from build123d import *

# Parameters (mm, degrees)
SZKIC1_R                    = 3
DODANIE_WYCI_GNI_CIE2_DEPTH = 2.4
SZKIC2_R                    = 1.5
DODANIE_WYCI_GNI_CIE3_DEPTH = 5
ZAOKR_GLENIE2_R             = 1.2
WYTNIJ_WYCI_GNI_CIE1_DEPTH  = 1.94


with BuildPart() as part:
    # Szkic1 → Dodanie-wyciągnięcie2 (new body)
    with BuildSketch(Plane.XY):
        with Locations((-1.860516246, 2.732142857)):
            Circle(SZKIC1_R)
    extrude(amount=DODANIE_WYCI_GNI_CIE2_DEPTH)

    # Szkic2 → Dodanie-wyciągnięcie3 (add)
    with BuildSketch(Plane(origin=(0, 0, 0), x_dir=(-1, 0, 0), z_dir=(0, 0, -1))):
        with Locations((1.860516246, 2.732142857)):
            Circle(SZKIC2_R)
    extrude(amount=DODANIE_WYCI_GNI_CIE3_DEPTH)

    # Zaokrąglenie2
    zaokr_glenie2_edges = [part.edges().sort_by_distance(p)[0] for p in [
        (-4.860516246, 2.732142857, 2.4),
    ]]
    fillet(zaokr_glenie2_edges, radius=ZAOKR_GLENIE2_R)

    # Szkic3 → Wytnij-wyciągnięcie1 (cut)
    with BuildSketch(Plane.XY.offset(2.4)):
        with BuildLine():
            Line((-1.859548318, 2.959091853), (-0.575649693, 5.316481314))
            ThreePointArc((-0.575649693, 5.316481314), (-0.297886623, 5.158637444), (-0.039271083, 4.97106076))
            Line((-0.039271083, 4.97106076), (-1.329373025, 2.669425378))
            Line((-1.329373025, 2.669425378), (-0.183967515, 2.043621837))
            ThreePointArc((-0.183967515, 2.043621837), (-0.320475658, 1.776553075), (-0.499159616, 1.535654258))
            Line((-0.499159616, 1.535654258), (-1.621312108, 2.148584891))
            Line((-1.621312108, 2.148584891), (-2.819933608, 0.01015725))
            ThreePointArc((-2.819933608, 0.01015725), (-3.083174674, 0.117799023), (-3.33454353, 0.250826496))
            Line((-3.33454353, 0.250826496), (-2.145142944, 2.434706401))
            Line((-2.145142944, 2.434706401), (-3.258687897, 3.042935511))
            ThreePointArc((-3.258687897, 3.042935511), (-3.162842423, 3.328316127), (-3.009463836, 3.587359481))
            Line((-3.009463836, 3.587359481), (-1.859548318, 2.959091853))
        make_face()
    extrude(amount=-WYTNIJ_WYCI_GNI_CIE1_DEPTH, mode=Mode.SUBTRACT)


solid = part.part
Geometry check sheet. Reference: the model listing, model coordinates, mm. A direction names the side the tool comes from. Give positions to 0.01 mm unless a question says otherwise; leave off trailing zeros. Write each loop counter-clockwise with the first axis right and the second up, starting at its lowest first coordinate (ties: lowest second). Pieces come first, ordered by that corner, then holes. Notation, with made-up numbers: M 36.5,14 L 63.5,14 A11 ccw 63.5,28 Z; hole C -39,45 d9. An arc over 180 degrees is marked long. One line per question, with ' | ' between items.
1. Scan lines: line 1 along X through (y, z) = (3.25, 1.5); line 2 along Y through (x, z) = (-0.75, 0.75); line 3 along Z through (x, y) = (-2.5, 1.5). Record each from-to range of solid material in increasing order. Write a range as from..to.
Ans:
line 1: -4.78..-3.2, -2.39..-1.7, -1..1.06 | line 2: -0.05..1.67, 2.35..3.7, 5..5.52 | line 3: -5..0.46
2. Cross-section at A-A (z = -3.75). Enter the section's corners in (x, y).
Ans:
outline: C -1.86,2.73 d3
3. Mould release check, pull along Y, two halves, no side actions. Record for faces 1 (the face through (-2, 3, -5)), 2 (the face through (-2.694, 2.735, 1.444)), 3 (the face through (-1.67, 4.22, -2.46)): released by +Y, released by -Y, zero draft, split by the parting line, or undercut.
Ans:
face 1: zero draft | face 2: undercut | face 3: split by the parting line
4. Set-up check for faces 4 (the face through (-1.227, 4.121, 1.444)), 5 (the face through (-3, 4, 0)), 6 (the face through (-2.7, 3.6, 2.4)): record each of +Z, -Z, +X, -X, +Y, -Y from which the full face is reachable in a straight line by a thin tool's end or side.
Ans:
face 4: +Z | face 5: -Z | face 6: +Z, +X, -X, +Y, -Y
5. Gauge pin test, flat end, axial feed: pin 1 (1 mm diameter, centred on x = -3.5, y = 5, fed in from -Z). Record the tip position at first contact, or that the pin passes through.
Ans:
pin 1: z = 0
